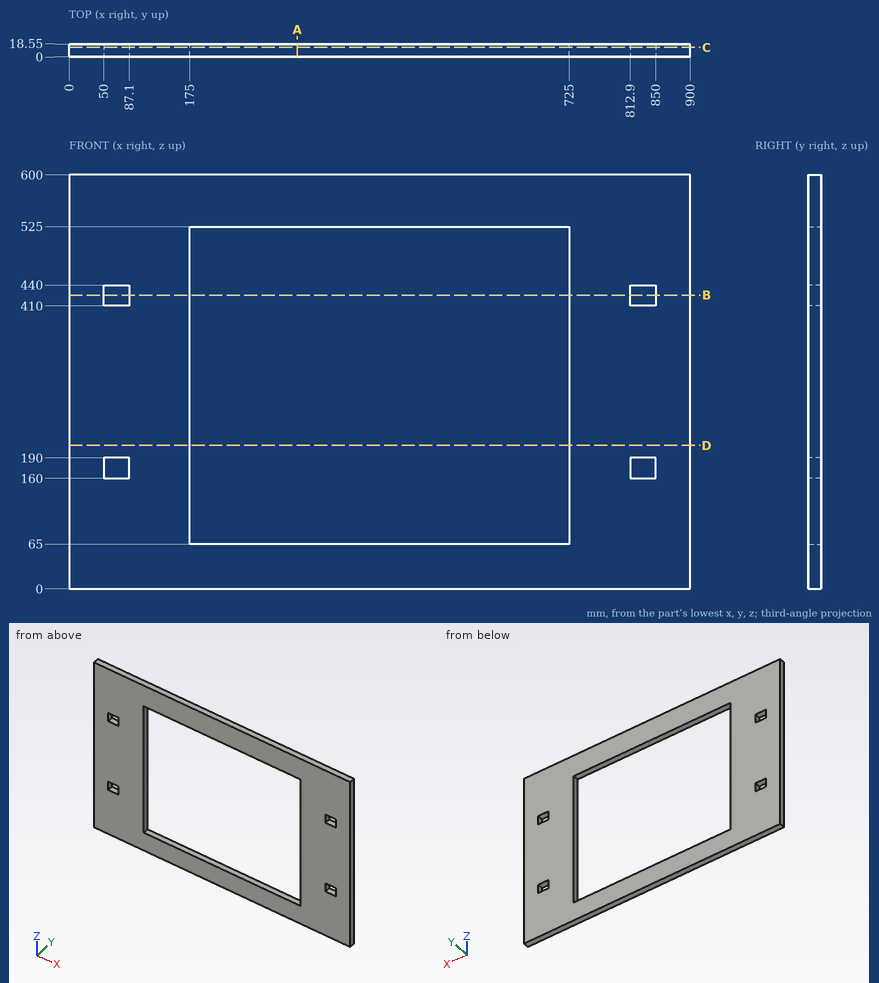
Source: three-view drawing plus pictorial views. Frame: mm from the lowest corner of the part. Round coordinates to 2 decimals unless told otherwise and drop trailing zeros. Write each loop counter-clockwise with the first axis right and the second up, starting at its lowest first coordinate (ties: lowest second). Pieces come first, ordered by that corner, then holes. Notation, with made-up numbers: M -39,19.25 L 0,19.25 A31 ccw 0,44.25 Z; hole C 50,60 d3. An arc over 180 degrees is marked long. Use CSV: the item, a comma, the result in double quotes. Start each with the question number.
Q1. Cut plane B-B on z = 425.5. Output: boundary loops of the cut face in (x, y).
Q2. Cut plane A-A on x = 331. Output: boundary loops of the cut face in (y, z), plus the area to 3 significant figures.
Q3. Cut plane D-D on z = 208. Output: boundary loops of the cut face in (x, y), plus the area to 3 significant figures.
Q4. Line query: line 1 (Z direction, x = 76.5, y = 14.75); line 2 (X direction, y = 16.5, z = 101.5); line 3 (Z direction, x = 570, y = 2). Output: solid intervals per line, ascending. Write a range as from..to.
Q5. Cut plane C-C on y = 13.75. Output: boundary loops of the cut face in (x, z), plus the area to 3 significant figures.
Results found:
1,outline,"M 0,0 L 50,0 L 50,18.55 L 0,18.55 Z; M 87.1,0 L 175,0 L 175,18.55 L 87.1,18.55 Z; M 725,0 L 812.9,0 L 812.9,18.55 L 725,18.55 Z; M 850,0 L 900,0 L 900,18.55 L 850,18.55 Z"
2,outline,"M 0,0 L 18.55,0 L 18.55,65 L 0,65 Z; M 0,525 L 18.55,525 L 18.55,600 L 0,600 Z"
2,area,"2,600 mm^2"
3,outline,"M 0,0 L 175,0 L 175,18.55 L 0,18.55 Z; M 725,0 L 900,0 L 900,18.55 L 725,18.55 Z"
3,area,"6,490 mm^2"
4,line 1,"0..160, 190..410, 440..600"
4,line 2,"0..175, 725..900"
4,line 3,"0..65, 525..600"
5,outline,"M 0,0 L 900,0 L 900,600 L 0,600 Z; hole M 50,160 L 87.1,160 L 87.1,190 L 50,190 Z; hole M 50,410 L 87.1,410 L 87.1,440 L 50,440 Z; hole M 175,65 L 725,65 L 725,525 L 175,525 Z; hole M 812.9,160 L 850,160 L 850,190 L 812.9,190 Z; hole M 812.9,410 L 850,410 L 850,440 L 812.9,440 Z"
5,area,"283,000 mm^2"
